```python
from build123d import *

# Parameters (mm, degrees)
FILLET1_R   = 0.4
FILLET2_R   = 0.8
HEX_2_DEPTH = 4


with BuildPart() as part:
    # BodySke → Base-Revolve (revolve)
    with BuildSketch(Plane.XY, mode=Mode.PRIVATE) as base_revolve_sk:
        Polygon((0, 0), (0, 6.5), (8, 6.5), (8, 4), (32.3095, 4), (33, 3.3095), (33, 0), align=None)
    revolve(base_revolve_sk.sketch.rotate(Axis((-31.75, 0, 0), (1, 0, 0)), 90), axis=Axis((-31.75, 0, 0), (1, 0, 0)))  # turned: the seam where the file's is

    # Fillet1
    fillet1_edges = [part.edges().sort_by_distance(p)[0] for p in [
        (8, 0, -4),
    ]]
    fillet(fillet1_edges, radius=FILLET1_R)

    # Fillet2
    fillet2_edges = [part.edges().sort_by_distance(p)[0] for p in [
        (0, 0, -6.5),
    ]]
    fillet(fillet2_edges, radius=FILLET2_R)

    # Sketch2 → Hex-PreBroach (revolve, cut)
    with BuildSketch(Plane.XY, mode=Mode.PRIVATE) as hex_prebroach_sk:
        Polygon((0, 3.01), (4, 3.01), (5.73782431, 0), (0, 0), align=None)
    revolve(hex_prebroach_sk.sketch.rotate(Axis((0, 0, 0), (1, 0, 0)), 90), axis=Axis((0, 0, 0), (1, 0, 0)), mode=Mode.SUBTRACT)  # turned: the seam where the file's is

    # Sketch3 → Hex 2 (cut)
    with BuildSketch(Plane(origin=(0, 0, 0), x_dir=(0, 0.5, 0.866025404), z_dir=(-1, 0, 0))):
        Polygon((1.73782431, 3.01), (-1.73782431, 3.01), (-3.475648621, 0), (-1.73782431, -3.01), (1.73782431, -3.01), (3.475648621, 0), align=None)
    extrude(amount=-HEX_2_DEPTH, mode=Mode.SUBTRACT)


solid = part.part
```
Verification items for the finished model (mm, model axes). A direction names the side the tool comes from. Give positions to 0.01 mm unless a question says otherwise; leave off trailing zeros. Order: outer loops, then holes, each group sorted by start corner. A loop starts at its lowest first (then second) coordinate and runs counter-clockwise, first axis right, second up. Notation, with made-up numbers: (45, 84) -> (72, 84) arc R24 cw to (72, 123) -> close; hole circle Ø3 at (-26.5, 71). An arc over 180 degrees is marked (long way). Use a Markdown table: item, result.
1) Section check A-A, the plane x = 29. Record the boundary of the cut face in (y, z), then the cut area to 3 significant figures.
Results:
| item | result |
|---|---|
| outline | circle Ø8 at (0, 0) |
| area | 50.3 mm² |
2) Tool access check on faces 4 (the cylindrical face through (4.45, 3.955, -5.158)), 5 (the flat face through (4, 1.5, 2.8)). Record the directions out of +Z, -Z, +X, -X, +Y, -Y that give a thin tool (end or side, any length) a straight path to the whole face; none if there is none.
Results:
| item | result |
|---|---|
| face 4 | +X, -X |
| face 5 | -X |
3) Mould release check, pull along Z, two halves, no side actions. Record for faces 1 (the flat face through (33, 0, 0)), 2 (the flat face through (4, 3.2, 0)), 3 (the cylindrical face through (20.522, 3.905, -0.867)): pulls with the +Z half, pulls with the -Z half, needs draft (parallel to the pull), parting line crosses it, or undercut.
Results:
| item | result |
|---|---|
| face 1 | needs draft |
| face 2 | undercut |
| face 3 | parting line crosses it |
4) Depth check by flat-ended pin: pin 1 Ø3 at (x, z) = (17.5, -1.5) entering from -Y; pin 2 Ø0.8 at (y, z) = (-1.5, 2) entering from -X; pin 3 Ø0.5 at (y, z) = (-1, -2.5) entering from -X. Enter the tip coordinate at first touch or a pass-through.
Results:
| item | result |
|---|---|
| pin 1 | y = -4 |
| pin 2 | x = 4.06 |
| pin 3 | x = 4.04 |
5) Material ranges on probe 1 along Y at (x, z) = (15, -2.25); probe 2 along X at (y, z) = (-5.5, -0.5); probe 3 along Z at (x, y) = (2, -0.25), recorded low to high.
Results:
| item | result |
|---|---|
| probe 1 | -3.31 to 3.31 |
| probe 2 | 0 to 8 |
| probe 3 | -6.5 to -3.01, 3.01 to 6.5 |
